```python
from build123d import *

# Parameters (mm, degrees)
BOSS_EXTRUDE1_DEPTH = 20.75
SKETCH2_R           = 7.3
BOSS_EXTRUDE2_DEPTH = 24.25
CUT_EXTRUDE1_DEPTH  = 50


with BuildPart() as part:
    # Sketch1 → Boss-Extrude1 (new body)
    with BuildSketch(Plane(origin=(0, 0, 0), x_dir=(1, 0, 0), z_dir=(0, 1, 0))):
        with BuildLine():
            Line((-2.3, -6.92820323), (-2.3, -9.601067812))
            Line((-2.3, -9.601067812), (2.3, -9.601067812))
            Line((2.3, -9.601067812), (2.3, -6.92820323))
            ThreePointArc((2.3, -6.92820323), (0, 7.3), (-2.3, -6.92820323))
        make_face()
    extrude(amount=BOSS_EXTRUDE1_DEPTH)

    # Sketch2 → Boss-Extrude2 (add)
    with BuildSketch(Plane(origin=(0, 20.75, 0), x_dir=(1, 0, 0), z_dir=(0, 1, 0))):
        with Locations(Location((0, 0, 0), (0, 0, 251.635051289))):
            Circle(SKETCH2_R)
    extrude(amount=BOSS_EXTRUDE2_DEPTH)

    # Sketch3 → Cut-Extrude1 (cut)
    with BuildSketch(Plane(origin=(0, 45, 0), x_dir=(1, 0, 0), z_dir=(0, 1, 0))):
        with BuildLine():
            Line((-2.5, 6.96491206), (2.5, 6.96491206))
            ThreePointArc((2.5, 6.96491206), (0, 7.4), (-2.5, 6.96491206))
        make_face()
    extrude(amount=-CUT_EXTRUDE1_DEPTH, mode=Mode.SUBTRACT)


solid = part.part
```
Here's how the part is built. I have some questions about the finished solid (model axes, mm). A direction names the side the tool comes from. Round coordinates to 2 decimals unless told otherwise and drop trailing zeros. Write each loop counter-clockwise with the first axis right and the second up, starting at its lowest first coordinate (ties: lowest second). Pieces come first, ordered by that corner, then holes. Notation, with made-up numbers: M -6.5,-13.75 L 15.5,-13.75 A21 ccw 15.5,22.25 Z; hole C 71.5,26.5 d6. An arc over 180 degrees is marked long. Answer as CSV lines item,"result". Start each with the question number.
1. Suppose I cut it at D-D on y = 26. Write out the boundary of the cut face in (x, z).
2. Suppose I cut it at B-B on z = 8.5. Write out the boundary of the cut face in (x, y), then the cut area to 4 significant figures.
3. I'm going to push flat-ended pins straight in: pin 1 Ø1.3 at (y, z) = (7.5, 8.5) entering from -X; pin 2 Ø2 at (y, z) = (7, 9) entering from +X; pin 3 Ø8 at (y, z) = (4.5, 5) entering from -X. Where does each tip first touch, or does it pass through?
4. Suppose I cut it at C-C on x = 0. Write out the boundary of the cut face in (y, z), then the cut area to 3 significant figures.
5. I need wall thicknesses on probe 1 along Z at (x, y) = (0, 31); probe 2 along X at (y, z) = (41.5, -0.25); probe 3 along X at (y, z) = (40, 5.5). Which ranges of each line are inside material? Lowest first, please.
6. On a 3-axis mill with a long thin cutter (end or side, diameter ignored), from which of +Z, -Z, +X, -X, +Y, -Y can I reach the whole of each face in a straight line? I mean faces 1 (the flat face through (-2.3, 10, 8)), 2 (the flat face through (0, 23, -6.965)), 3 (the flat face through (2.3, 10, 8)). Say none if no direction works.
7. Suppose I cut it at A-A on y = 9. Write out the boundary of the cut face in (x, z).
Check result:
1,outline,"M -2.19,-6.96 L 2.19,-6.96 A7.3 ccw long Z"
2,outline,"M -2.3,0 L 2.3,0 L 2.3,20.75 L -2.3,20.75 Z"
2,area,"95.45 mm2"
3,pin 1,"stops at x = -2.3"
3,pin 2,"stops at x = 2.3"
3,pin 3,"stops at x = -7.23"
4,outline,"M 0,-6.96 L 45,-6.96 L 45,7.3 L 20.75,7.3 L 20.75,9.6 L 0,9.6 Z"
4,area,"690 mm2"
5,probe 1,"z = -6.96 to 7.3"
5,probe 2,"x = -7.3 to 7.3"
5,probe 3,"x = -4.8 to 4.8"
6,face 1,"+Z, -X, +Y, -Y"
6,face 2,"-Z, +X, -X, +Y, -Y"
6,face 3,"+Z, +X, +Y, -Y"
7,outline,"M -2.3,6.93 A7.3 ccw -2.19,-6.96 L 2.19,-6.96 A7.3 ccw 2.3,6.93 L 2.3,9.6 L -2.3,9.6 Z"
